Could you check a few things on this model? Use its own coordinates, in mm. A direction names the side the tool comes from. Coordinates: 2 decimals unless noted, no trailing zeros. Loops run counter-clockwise (first coordinate to the right, second up) from the corner with the lowest first, then second, coordinate; pieces in that order, holes last. Notation, with made-up numbers: (-31, -28) -> (-3, -28) arc R19 cw to (-3, -4) -> close; hole circle Ø9 at (77.25, -38.75). An arc over 180 degrees is marked (long way). One line per question, with ' | ' between items. Start each with the question number.
(1) Suppose I cut it at B-B (y = 0). Give the number of separate pieces and of enclosed holes in the cut face, plus the area to 3 significant figures.
(2) Suppose I cut it at A-A (x = 0). Please give me the cut outline in (y, z).
(3) I'm going to push flat-ended pins straight in: pin 1 Ø20 at (x, z) = (0, 18.1) entering from -Y; pin 2 Ø12.5 at (x, z) = (5, 16.5) entering from +Y; pin 3 Ø9.5 at (x, y) = (-25, -1.5) entering from +Z. Where does each tip first touch, or does it pass through?
(4) If we mould it in two halves opening along Y, with no side actions, what happens to faces 1 (the face through (0, 10, 5)), 2 (the face through (-1, 0, 23)), 3 (the face through (-17.85, 1.62, 23.63)), 4 (the face through (-26.3, -0.1, 7.2))? For each: pulls with the +Y half, pulls with the -Y half, needs draft (parallel to the pull), parting line crosses it, or undercut.
(5) If I drill on line 1 along X through (y, z) = (-3, 0); line 2 along X through (y, z) = (-0.25, 7); line 3 along Z through (x, y) = (-23, -7.75), over which ranges is the centre line in solid material (lowest first)?
(6) Suppose I cut it at C-C (x = -23). Please give me the cut outline in (y, z).
(7) Which directions (+Z, -Z, +X, -X, +Y, -Y) give clear straight access to the entire face, cutting with the end or side of a thin tool? Please do faces 5 (the face through (-17, 0, 30)), 6 (the face through (-2.71, -8.73, 5.9)), 7 (the face through (-23, -4, 21.603)).
(8) Suppose I cut it at D-D (z = 33). Please give me the cut outline in (x, y), plus the area to 3 significant figures.
```python
from build123d import *

# Parameters (mm, degrees)
F0_R     = 2.75
F0_R_2   = 12.5
F1_DEPTH = 10
F0_R_3   = 5
F2_DEPTH = 7.5
F3_SIZE  = 2
F4_R     = 1
F5_R     = 3.3
F6_DEPTH = 32.5
F7_R     = 5.4
F7_R_2   = 3.3
F8_DEPTH = 4


with BuildPart() as f1:
    # F0 (on Front) → F1 (new body, symmetric)
    with BuildSketch(Plane.XZ):
        Polygon((-17, 25.6028276384), (-30, 25.6028276384), (-30, -6.8971723616), (30, -6.8971723616), (30, 25.6028276384), (17, 25.6028276384), (17, 36.1028276384), (-17, 36.1028276384), align=None)
        with Locations((-23, 0.1028276384)):
            Circle(F0_R, mode=Mode.SUBTRACT)
        with Locations((23, 0.1028276384)):
            Circle(F0_R, mode=Mode.SUBTRACT)
        with Locations((-23, 18.1028276384)):
            Circle(F0_R, mode=Mode.SUBTRACT)
        with Locations((0, 18.1028276384)):
            Circle(F0_R_2, mode=Mode.SUBTRACT)
        with Locations((23, 18.1028276384)):
            Circle(F0_R, mode=Mode.SUBTRACT)
    extrude(amount=F1_DEPTH, both=True)

    # F0 (on Front) → F2 (join, symmetric)
    with BuildSketch(Plane.XZ):
        with Locations((0, 18.1028276384)):
            Circle(F0_R_2)
        with Locations((0, 18.1028276384)):
            Circle(F0_R_3, mode=Mode.SUBTRACT)
    extrude(amount=F2_DEPTH, both=True)

    # F3
    f3_edges = [f1.edges().sort_by_distance(p)[0] for p in [
        (-17, 0, 36.102828),
        (17, 0, 36.102828),
    ]]
    chamfer(f3_edges, length=F3_SIZE)

    # F4
    f4_edges = [f1.edges().sort_by_distance(p)[0] for p in [
        (-30, 0, 25.602828),
        (30, 0, 25.602828),
    ]]
    fillet(f4_edges, radius=F4_R)

    # F5 (on face) → F6 (cut)
    with BuildSketch(Plane(origin=(0, 0, -6.8971723616), x_dir=(1, 0, 0), z_dir=(0, 0, -1))):
        with Locations((23, 0)):
            Circle(F5_R)
        with Locations((-23, 0)):
            Circle(F5_R)
    extrude(amount=-F6_DEPTH, mode=Mode.SUBTRACT)

    # F7 (on face) → F8 (cut)
    with BuildSketch(Plane.XY.offset(25.6028276384)):
        with Locations((23, 0)):
            Circle(F7_R)
        with Locations((23, 0)):
            Circle(F7_R_2, mode=Mode.SUBTRACT)
        with Locations((-23, 0)):
            Circle(F7_R)
    extrude(amount=-F8_DEPTH, mode=Mode.SUBTRACT)


solid = f1.part
```
Checks:
1) separate pieces: 3 | enclosed holes: 1 | area: 1,760 mm^2
2) outline: (-10, -6.9) -> (10, -6.9) -> (10, 5.6) -> (7.5, 5.6) -> (7.5, 13.1) -> (-7.5, 13.1) -> (-7.5, 5.6) -> (-10, 5.6) -> close; (-10, 30.6) -> (-7.5, 30.6) -> (-7.5, 23.1) -> (7.5, 23.1) -> (7.5, 30.6) -> (10, 30.6) -> (10, 36.1) -> (-10, 36.1) -> close
3) pin 1: stops at y = -7.5 | pin 2: stops at y = 7.5 | pin 3: stops at z = 25.6
4) face 1: pulls with the +Y half | face 2: needs draft | face 3: undercut | face 4: undercut
5) line 1: x = -30 to -25.75, -20.25 to 20.25, 25.75 to 30 | line 2: x = -30 to -26.29, -19.71 to 19.71, 26.29 to 30 | line 3: z = -6.9 to -2.65, 2.85 to 15.35, 20.85 to 25.6
6) outline: (-10, -6.9) -> (-3.3, -6.9) -> (-3.3, -2.65) -> (-10, -2.65) -> close; (-10, 2.85) -> (-3.3, 2.85) -> (-3.3, 15.35) -> (-10, 15.35) -> close; (-10, 20.85) -> (-3.3, 20.85) -> (-3.3, 21.6) -> (-5.4, 21.6) -> (-5.4, 25.6) -> (-10, 25.6) -> close; (3.3, -6.9) -> (10, -6.9) -> (10, -2.65) -> (3.3, -2.65) -> close; (3.3, 2.85) -> (10, 2.85) -> (10, 15.35) -> (3.3, 15.35) -> close; (3.3, 20.85) -> (10, 20.85) -> (10, 25.6) -> (5.4, 25.6) -> (5.4, 21.6) -> (3.3, 21.6) -> close
7) face 5: +Z, -X, +Y, -Y | face 6: -Y | face 7: +Z
8) outline: (-17, -10) -> (17, -10) -> (17, 10) -> (-17, 10) -> close | area: 680 mm^2
